Autodesk Inventor part; units mm, degrees
ref_plane "YZ Plane" through (0, 0, 0) normal (1, 0, 0) x (0, 1, 0)
ref_plane "XZ Plane" through (0, 0, 0) normal (0, 1, 0) x (-1, 0, 0)
ref_plane "XY Plane" through (0, 0, 0) normal (0, 0, 1) x (1, 0, 0)
sketch "Sketch1" plane through (0, 0, 0) normal (0, 0, 1) x (1, 0, 0)
  circle A0 centre (0, 0) radius 15
  circle A1 centre (-12.5, 0) radius 1.4
  circle A2 centre (0, -12.5) radius 1.4
  circle A3 centre (12.5, 0) radius 1.4
  circle A4 centre (0, 12.5) radius 1.4
  arc A5 (139.8092, 1.0191) -> (139.8092, -1.0191) centre (150, 0) ccw
  line L0 (0, 15) -> (150, 0)
  line L1 (0, -15) -> (150, 0)
  line L2 (29.7634, 10.0809) -> (35.7634, 10.0809)
  line L3 (35.7634, 10.0809) -> (35.7634, -10.0809)
  line L4 (35.7634, -10.0809) -> (29.7634, -10.0809)
  line L5 (29.7634, -10.0809) -> (29.7634, 10.0809)
  line L6 (29.7634, 10.0809) -> (35.7634, -10.0809) construction
  line L7 (35.7634, 10.0809) -> (29.7634, -10.0809) construction
  line L8 (38.7634, 10.0809) -> (44.7634, 10.0809)
  line L9 (44.7634, 10.0809) -> (44.7634, -10.0809)
  line L10 (44.7634, -10.0809) -> (38.7634, -10.0809)
  line L11 (38.7634, -10.0809) -> (38.7634, 10.0809)
  line L12 (38.7634, 10.0809) -> (44.7634, -10.0809) construction
  line L13 (44.7634, 10.0809) -> (38.7634, -10.0809) construction
  line L14 (47.7634, 8.546) -> (53.7634, 8.546)
  line L15 (53.7634, 8.546) -> (53.7634, -8.546)
  line L16 (53.7634, -8.546) -> (47.7634, -8.546)
  line L17 (47.7634, -8.546) -> (47.7634, 8.546)
  line L18 (47.7634, 8.546) -> (53.7634, -8.546) construction
  line L19 (53.7634, 8.546) -> (47.7634, -8.546) construction
  line L20 (62.7634, 7.5) -> (56.7634, 7.5)
  line L21 (56.7634, 7.5) -> (56.7634, -7.5)
  line L22 (56.7634, -7.5) -> (62.7634, -7.5)
  line L23 (62.7634, -7.5) -> (62.7634, 7.5)
  line L24 (62.7634, 7.5) -> (56.7634, -7.5) construction
  line L25 (56.7634, 7.5) -> (62.7634, -7.5) construction
  line L26 (71.7634, 6.9773) -> (65.7634, 6.9773)
  line L27 (65.7634, 6.9773) -> (65.7634, -6.9773)
  line L28 (65.7634, -6.9773) -> (71.7634, -6.9773)
  line L29 (71.7634, -6.9773) -> (71.7634, 6.9773)
  line L30 (71.7634, 6.9773) -> (65.7634, -6.9773) construction
  line L31 (65.7634, 6.9773) -> (71.7634, -6.9773) construction
  line L32 (20.7634, 11) -> (26.7634, 11)
  line L33 (26.7634, 11) -> (26.7634, -11)
  line L34 (26.7634, -11) -> (20.7634, -11)
  line L35 (20.7634, -11) -> (20.7634, 11)
  line L36 (20.7634, 11) -> (26.7634, -11) construction
  line L37 (26.7634, 11) -> (20.7634, -11) construction
  line L38 (20.7634, 11) -> (26.7634, 0)
  line L39 (20.7634, -11) -> (26.7634, 0)
  line L40 (29.7634, 10.0809) -> (35.7634, 0)
  line L41 (29.7634, -10.0809) -> (35.7634, 0)
  line L42 (38.7634, 10.0809) -> (44.7634, 0)
  line L43 (38.7634, -10.0809) -> (44.7634, 0)
  line L44 (47.7634, 8.546) -> (53.7634, 0)
  line L45 (47.7634, -8.546) -> (53.7634, 0)
  line L46 (56.7634, 7.5) -> (62.7634, 0)
  line L47 (56.7634, -7.5) -> (62.7634, 0)
  line L48 (65.7634, 6.9773) -> (71.7634, 0)
  line L49 (65.7634, -6.9773) -> (71.7634, 0)
  line L50 (78.7015, 4.273) -> (78.7015, -5.0405)
  line L51 (78.7015, -5.0405) -> (98.1361, -0.3837)
  line L52 (98.1361, -0.3837) -> (78.7015, 4.273)
  point P0 (32.7634, 0)
  point P1 (41.7634, 0)
  point P2 (50.7634, 0)
  point P3 (59.7634, 0)
  point P4 (68.7634, 0)
  point P5 (23.7634, 0)
  dimension "d0" = 30
  dimension "d1" = 2.8
  dimension "d2" = 12.5
  dimension "d5" = 360
  dimension "d7" = 150
  dimension "d8" = 9
  dimension "d9" = 9
  dimension "d10" = 9
  dimension "d11" = 9
  dimension "d12" = 6
  dimension "d13" = 6
  dimension "d14" = 6
  dimension "d15" = 6
  dimension "d16" = 6
  dimension "d17" = 6
  dimension "d18" = 9
  dimension "d19" = 22
extrude "Extrusion1" add sketch "Sketch1" along normal blind 3 contours L0 A0 L1 | L0 A5 L1 A0 | L0 L1 A5 | L2 L3 L40 | L41 L3 L4 | L8 L9 L42 | L43 L9 L10 | L14 L15 L44 | L45 L15 L16 | L23 L46 L20 | L23 L22 L47 | L29 L48 L26 | L29 L28 L49 | L32 L33 L38 | L39 L33 L34
sketch "Sketch2" plane through (0, 0, 3) normal (0, 0, 1) x (1, 0, 0)
  circle A0 centre (0, 0) radius 1.5
  dimension "d22" = 3
extrude "Extrusion2" cut sketch "Sketch2" against normal through all
properties part number "link2"
Read the model definition and answer for the solid it produces. Units are mm, in the model's axes. A direction names the side the tool comes from. Coordinates: 2 decimals unless noted, no trailing zeros. Order: outer loops, then holes, each group sorted by start corner. A loop starts at its lowest first (then second) coordinate and runs counter-clockwise, first axis right, second up. Notation, with made-up numbers: (-25.5, 69.25) - (1.5, 69.25) arc R34 cw to (1.5, 106.25) - close; hole circle Ø9 at (55.25, 21.5). An arc over 180 degrees is marked (long way). Answer as a JSON object with one key per item and string values. Group by question number.
Item 1: Section A-A (z = 1.75) is taken. State how many separate pieces and enclosed holes the cut face has, plus the area to 3 significant figures.
Item 2: A flat-ended cylindrical pin translates along its axis: P1, Ø1.5, axis at x = 117.5, z = 2.5, coming from the -Y side (3 decimals). Find the tip coordinate at first contact, or state that the pin passes through.
Item 3: Consider probe 1 along Y at (x, z) = (0, 2.1); probe 2 along Y at (x, z) = (0.5, 0.85); probe 3 along Y at (x, z) = (24, 2.3). Determine where each line is inside the solid, lowest interval first. Write a range as from..to.
Item 4: The mould has two halves that part along X. Classify faces 3 (the face through (88.6, 1.9, 1.5)), 4 (the face through (30, -10, 0)), 5 (the face through (59.721, -3.803, 1.479)), 6 (the face through (74, -7.6, 1.5)): +X half, -X half, draft (parallel to the pull), parting line (faces both ways), or undercut.
Item 5: Section D-D (y = -12.5) is taken. Give the vertices of the cut face in (x, z), plus the area to 3 significant figures.
Item 6: Section B-B (x = 12.5) is taken. Give the vertices of the cut face in (y, z), plus the area to 3 significant figures.
Item 7: A tool of negligible diameter and unlimited length cuts with its end or side. For faces 1 (the face through (30, -10, 3)), 2 (the face through (20.763, 0, 1)), from which of +Z, -Z, +X, -X, +Y, -Y can it reach the whole face along a straight path? Write none if from no direction.
Results are:
{
 "1": {"separate pieces": "1", "enclosed holes": "12", "area": "2,160 mm^2"},
 "2": {"P1": "stops at y = -3.325"},
 "3": {"probe 1": "y = -15..-13.9, -11.1..-1.5, 1.5..11.1, 13.9..15", "probe 2": "y = -14.95..-13.81, -11.19..-1.41, 1.41..11.19, 13.81..14.95", "probe 3": "y = -12.6..-5.07, 5.07..12.6"},
 "4": {"face 3": "undercut", "face 4": "draft", "face 5": "undercut", "face 6": "+X half"},
 "5": {"outline": "(-8.29, 0) - (-1.4, 0) - (-1.4, 3) - (-8.29, 3) - close; (1.4, 0) - (25, 0) - (25, 3) - (1.4, 3) - close", "area": "91.5 mm^2"},
 "6": {"outline": "(-13.75, 0) - (-1.4, 0) - (-1.4, 3) - (-13.75, 3) - close; (1.4, 0) - (13.75, 0) - (13.75, 3) - (1.4, 3) - close", "area": "74.1 mm^2"},
 "7": {"face 1": "+Z, +X, -X, +Y, -Y", "face 2": "+Z, -Z"}
}
